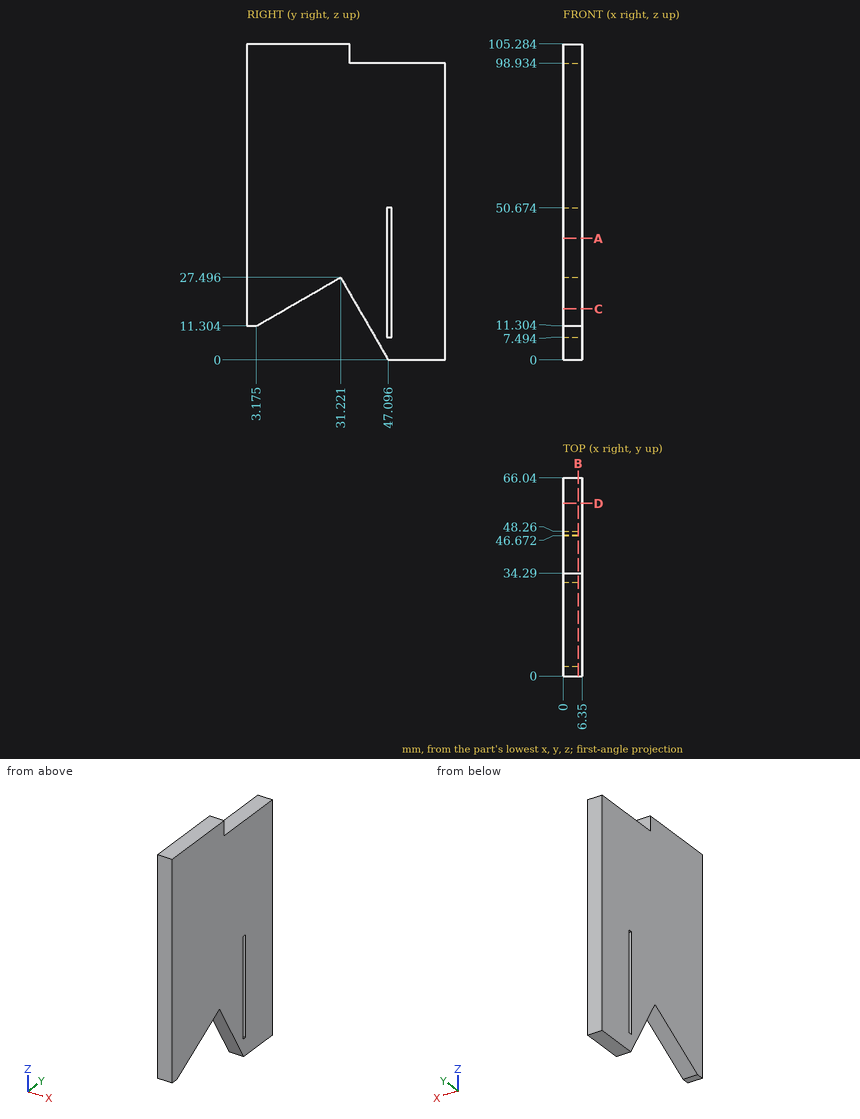
The figure shows three views and two pictorial views of one solid part (mm, origin at its lowest corner). Answer the questions. Give positions to 0.01 mm unless a question says otherwise; leave off trailing zeros. Order: outer loops, then holes, each group sorted by start corner. A loop starts at its lowest first (then second) coordinate and runs counter-clockwise, first axis right, second up. Notation, with made-up numbers: M -13.5,49 L 6.5,49 A30 cw 6.5,79 Z; hole C 11.5,21.25 d11. An arc over 180 degrees is marked long. Return JSON: item names as keys, results as strings.
1) Section A-A, the plane z = 40.5 is taken. Write down the section's boundary in (x, y).
Resolved:
{"outline": "M 0,0 L 6.35,0 L 6.35,46.67 L 0,46.67 Z; M 0,48.26 L 6.35,48.26 L 6.35,66.04 L 0,66.04 Z"}
2) Straight lines are drawn through the part: line 1 along Y through (x, z) = (4.25, 50); line 2 along Y through (x, z) = (1.25, 16) (1 decimal); line 3 along Y through (x, z) = (1, 15) (1 decimal). For each, find the intervals that lie inside material, in ascending order. Write a range as [from, to].
Resolved:
{"line 1": "[0, 46.67], [48.26, 66.04]", "line 2": "[0, 11.3], [37.9, 46.7], [48.3, 66]", "line 3": "[0, 9.6], [38.4, 46.7], [48.3, 66]"}
3) Section D-D, the plane y = 57.5 is taken. Write down the section's boundary in (x, z), plus the area to 3 significant figures.
Resolved:
{"outline": "M 0,0 L 6.35,0 L 6.35,98.93 L 0,98.93 Z", "area": "628 mm^2"}
4) Section B-B, the plane x = 5 is taken. Write down the section's boundary in (y, z) (1 decimal).
Resolved:
{"outline": "M 0,11.3 L 3.2,11.3 L 31.2,27.5 L 47.1,0 L 66,0 L 66,98.9 L 34.3,98.9 L 34.3,105.3 L 0,105.3 Z; hole M 46.7,7.5 L 48.3,7.5 L 48.3,50.7 L 46.7,50.7 Z"}
5) Section C-C, the plane z = 17 is taken. Write down the section's boundary in (x, y), plus the area to 3 significant figures.
Resolved:
{"outline": "M 0,0 L 6.35,0 L 6.35,13.04 L 0,13.04 Z; M 0,37.28 L 6.35,37.28 L 6.35,46.67 L 0,46.67 Z; M 0,48.26 L 6.35,48.26 L 6.35,66.04 L 0,66.04 Z", "area": "255 mm^2"}
6) Each of these flat-tipped pins is pushed along its axis until it touches: pin 1 (1 mm diameter, centred on x = 2, z = 73, fed in from -Y); pin 2 (2 mm diameter, centred on x = 3.5, y = 10, fed in from -Z); pin 3 (1 mm diameter, centred on x = 4, y = 10.5, fed in from -Z) (1 decimal); pin 4 (1.9 mm diameter, centred on x = 4, y = 43.5, fed in from +Z). Where does it stop, or does it pass through?
Resolved:
{"pin 1": "y = 0", "pin 2": "z = 14.67", "pin 3": "z = 15.2", "pin 4": "z = 98.93"}
